Part print with two shaded views. Sizes in mm from the minimum x, y, z corner. Coordinates: 2 decimals unless noted, no trailing zeros. Loops run counter-clockwise (first coordinate to the right, second up) from the corner with the lowest first, then second, coordinate; pieces in that order, holes last.
Item 1: Drill centre lines: line 1 along X through (y, z) = (5.25, 2); line 2 along Y through (x, z) = (14.5, 2.5); line 3 along X through (y, z) = (4, 4) (3 decimals). Where is each one in solid material? Low to high.
Item 2: Cut at C-C (x = 11). List the corners of the cut face in (y, z), and give its area (3 significant figures).
Item 3: Cut at D-D (x = 16.5). List the corners of the cut face in (y, z).
Item 4: Cut at A-A (z = 3.25). List the corners of the cut face in (x, y).
Item 5: Mould opens along X. For the marked faces 1, 2 and 3 say: released by +X, released by -X, zero draft, split by the parting line, or undercut.
Item 6: Flat gauge pins, fed straight in: pin 1 (1 mm diameter, centred on y = 3, z = 2.5, fed in from -X); pin 2 (1.5 mm diameter, centred on x = 8, z = 3, fed in from +Y); pin 3 (1.5 mm diameter, centred on x = 11, z = 2.5, fed in from -Y). Where does each tip first touch, or does it go through?
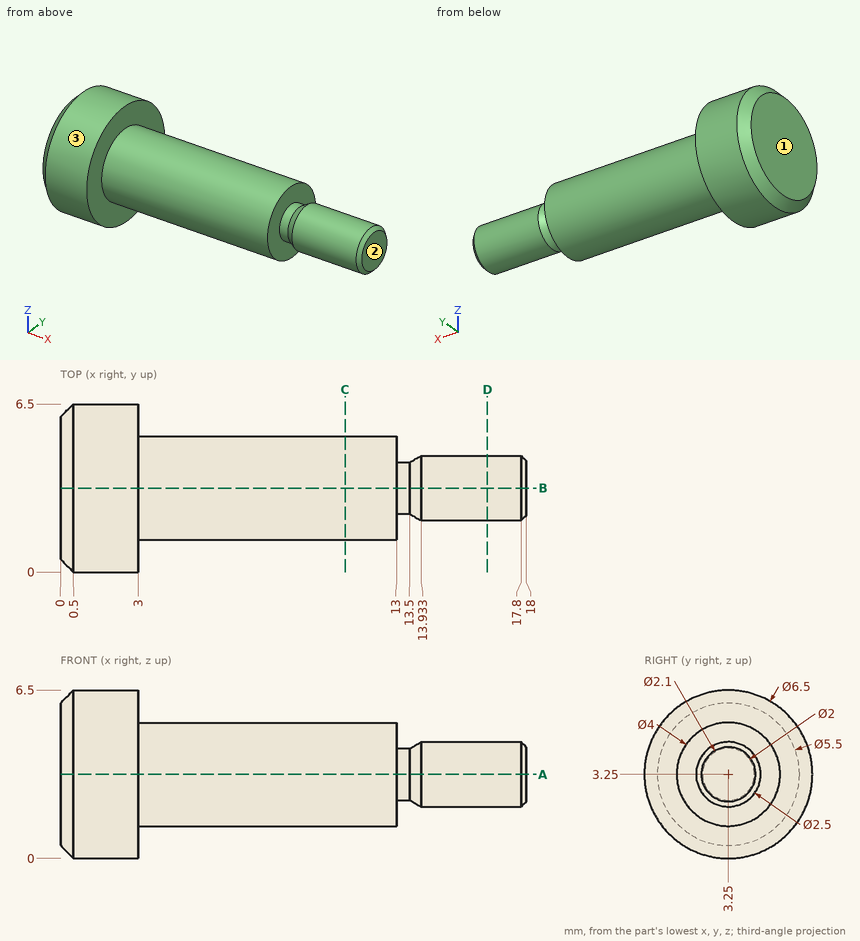
Filled sheet:
1. line 1: x = 0 to 3
1. line 2: y = 2.25 to 4.25
1. line 3: x = 0 to 13, 13.605 to 17.989
2. outline: circle Ø4 at (3.25, 3.25)
2. area: 12.6 mm2
3. outline: circle Ø2.5 at (3.25, 3.25)
4. outline: (0, 0.5) - (0.5, 0) - (3, 0) - (3, 1.25) - (13, 1.25) - (13, 2.25) - (13.5, 2.25) - (13.93, 2) - (17.8, 2) - (18, 2.2) - (18, 4.3) - (17.8, 4.5) - (13.93, 4.5) - (13.5, 4.25) - (13, 4.25) - (13, 5.25) - (3, 5.25) - (3, 6.5) - (0.5, 6.5) - (0, 6) - close
5. face 1: released by -X
5. face 2: released by +X
5. face 3: zero draft
6. pin 1: stops at x = 0
6. pin 2: stops at y = 5.25
6. pin 3: stops at y = 1.25
